The listing builds one solid part. Answer for the finished solid, in the listing's coordinates (mm). A direction names the side the tool comes from. Round coordinates to 2 decimals unless told otherwise and drop trailing zeros. Order: outer loops, then holes, each group sorted by start corner. A loop starts at its lowest first (then second) coordinate and runs counter-clockwise, first axis right, second up. Notation, with made-up numbers: M 63,43.5 L 114,43.5 A20 cw 114,67.5 Z; hole C -5,-39 d4. An arc over 180 degrees is marked long. Write item = value, one per line. Start each with the question number.
(1) Straight lines are drawn through the part: probe 1 along Z at (x, y) = (-21, -13.5); probe 2 along X at (y, z) = (-14, 9.5); probe 3 along Z at (x, y) = (15, -19). For each, find the intervals that lie inside material, in ascending order. Write a range as from..to.
(2) For a pull along X with two mould halves and no side action, classify faces 5 (the face through (-55.976, -13, -36)), 6 (the face through (-3, -13, -17.575)), 7 (the face through (-47, -13, -17.575)) as released by +X, released by -X, zero draft, split by the parting line, or undercut.
(3) A cutting plane is placed at A-A, the plane x = 26. Determine the outline of the cut face in (y, z), and give its area (3 significant figures).
(4) Each of these flat-tipped pins is pushed along its axis until it touches: pin 1 (7.5 mm diameter, centred on x = 6, y = -11, fed in from +Z); pin 2 (12.5 mm diameter, centred on y = -19, z = -33.5, fed in from +X); pin 3 (10 mm diameter, centred on y = -3.5, z = -5.5, fed in from +X); pin 4 (1.5 mm diameter, centred on x = -14.5, z = 15.5, fed in from +Y). Where does it stop, or does it pass through?
(5) Which of the six approach directions +Z, -Z, +X, -X, +Y, -Y give full straight-line access (tool end or side, diameter ignored) to faces 1 (the face through (-41.773, -12.522, 42.365)), 2 (the face through (60.69, -13, -37)), 3 (the face through (57, -13, 53.181)), 4 (the face through (25.73, -12.52, -24.73))?
(6) A cutting plane is placed at C-C, the plane z = 34. Determine the outline of the cut face in (x, y).
(7) A cutting plane is placed at D-D, the plane x = -44. Determine the outline of the cut face in (y, z).
(8) A cutting plane is placed at B-B, the plane y = -16. Determine the outline of the cut face in (x, z).
from build123d import *

# Parameters (mm, degrees)
F1_DEPTH = 25.4


with BuildPart() as f1:
    # F0 (on Front) → F1 (new body)
    with BuildSketch(Plane.XZ):
        Polygon((-33.9528769255, 40.0564680563), (-33.9528769255, 53.1810894608), (18.2133984662, 53.1810894608), (51.5383630991, 65.2996533445), (51.5383630991, 66.3159769478), (13.3911538869, 86.7411494255), (-49.376770854, 44.6101650596), align=None)
        Polygon((18.2133984662, 53.1810894608), (-33.9528769255, 53.1810894608), (-33.9528769255, 40.0564680563), (-15.8423800021, 34.7095876932), (-14.4241497444, 34.3657573582), (45.7716546953, 19.7721160948), (28.9523048901, -17.5747666508), (51.5383630991, -17.5747666508), (51.5383630991, 53.1810894608), align=None)
        Polygon((51.5383630991, 65.2996533445), (18.2133984662, 53.1810894608), (51.5383630991, 53.1810894608), align=None)
        Polygon((-15.8423800021, 34.7095876932), (-33.9528769255, 40.0564680563), (-33.9528769255, -7.1603319994), (-14.4241497444, 34.3657573582), align=None)
        Polygon((51.5383630991, 65.2996533445), (51.5383630991, 53.1810894608), (62.3221695423, 53.1810894608), (62.3221695423, 72.0649734139), (51.5383630991, 72.0649734139), (51.5383630991, 66.3159769478), (52.6687689126, 65.7107234001), align=None)
        Polygon((51.5383630991, 66.3159769478), (51.5383630991, 65.2996533445), (52.6687689126, 65.7107234001), align=None)
        Polygon((-14.4241497444, 34.3657573582), (-33.9528769255, -7.1603319994), (-33.9528769255, -17.5747666508), (28.9523048901, -17.5747666508), (45.7716546953, 19.7721160948), align=None)
        Polygon((-33.9528769255, -17.5747666508), (-33.9528769255, -7.1603319994), (-38.8505365943, -17.5747666508), align=None)
        Polygon((60.6898404658, -17.5747666508), (51.5383630991, -17.5747666508), (51.5383630991, -32.0976935327), (22.4118343216, -32.0976935327), (15.7569888979, -46.8745864928), (-47.0071732998, -34.9191240966), (-38.8505365943, -17.5747666508), (-55.9755302966, -17.5747666508), (-55.9755302966, -55.0077706575), (60.6898404658, -55.0077706575), align=None)
        Polygon((51.5383630991, -32.0976935327), (51.5383630991, -17.5747666508), (28.9523048901, -17.5747666508), (22.4118343216, -32.0976935327), align=None)
        Polygon((-33.9528769255, -32.0976935327), (-33.9528769255, -17.5747666508), (-38.8505365943, -17.5747666508), (-47.0071732998, -34.9191240966), (15.7569888979, -46.8745864928), (22.4118343216, -32.0976935327), align=None)
    extrude(amount=F1_DEPTH)


solid = f1.part
Reported:
q1.probe_1 = -55.01..-32.1, -17.57..63.66
q1.probe_2 = -33.95..51.54
q1.probe_3 = -55.01..-32.1, -17.57..85.88
q2.face_5 = released by -X
q2.face_6 = undercut
q2.face_7 = zero draft
q3.outline = M -25.4,-55.01 L 0,-55.01 L 0,-24.13 L -25.4,-24.13 Z; M -25.4,-17.57 L 0,-17.57 L 0,79.99 L -25.4,79.99 Z
q3.area = 3,260 mm²
q4.pin_1 = 84.3
q4.pin_2 = 60.69
q4.pin_3 = 51.54
q4.pin_4 = 0
q5.face_1 = -X, +Y, -Y
q5.face_2 = -Z, +X, +Y, -Y
q5.face_3 = +X, +Y, -Y
q5.face_4 = +Y, -Y
q6.outline = M -33.95,-25.4 L 51.54,-25.4 L 51.54,0 L -33.95,0 Z
q7.outline = M -25.4,-55.01 L 0,-55.01 L 0,-17.57 L -25.4,-17.57 Z; M -25.4,43.02 L 0,43.02 L 0,48.22 L -25.4,48.22 Z
q8.outline = M -55.98,-55.01 L 60.69,-55.01 L 60.69,-17.57 L 51.54,-17.57 L 51.54,53.18 L 62.32,53.18 L 62.32,72.06 L 51.54,72.06 L 51.54,66.32 L 13.39,86.74 L -49.38,44.61 L -33.95,40.06 L -33.95,-7.16 L -38.85,-17.57 L -55.98,-17.57 Z; hole M -33.95,-32.1 L 22.41,-32.1 L 28.95,-17.57 L -33.95,-17.57 Z
